Job drawing, mm, ordinate dimensions from the low corner. One solid piece. A direction names the side the tool comes from. Round coordinates to 2 decimals unless told otherwise and drop trailing zeros. Loops run counter-clockwise (first coordinate to the right, second up) from the corner with the lowest first, then second, coordinate; pieces in that order, holes last.
1) Band-saw the part on A-A, the plane x = 210. Write the cut outline in (y, z).
2) Drop flat-ended pins along their axis: P1, Ø1.5, axis at y = 9.5, z = 34, coming from the +X side; P2, Ø6, axis at x = 28, y = 4.5, coming from the +Z side; P3, Ø6, axis at x = 200.5, y = 13, coming from the -Z side. Give the stop position or say it passes through.
3) 3-axis set-ups, long thin cutter, end or side, ignore diameter. For the marked faces 4, 5 and 6: which of +Z, -Z, +X, -X, +Y, -Y reach the whole face in a straight line?
4) Band-saw the part on B-B, the plane y = 14.5. Write the cut outline in (x, z), then the cut area to 3 significant figures.
5) Band-saw the part on C-C, the plane z = 45. Write the cut outline in (x, y), then the cut area to 3 significant figures.
6) Probe line 1 (Z direction, x = 102, y = 11.5); line 2 (Z direction, x = 45, y = 10); line 3 (X direction, y = 13.25, z = 45). List the from-to ranges inside material, lowest first.
7) Mould opens along X. For the marked faces 1, 2 and 3 say: +X half, -X half, draft (parallel to the pull), parting line (faces both ways), or undercut.
8) Band-saw the part on D-D, the plane x = 45. Write the cut outline in (y, z), then the cut area to 3 significant figures.
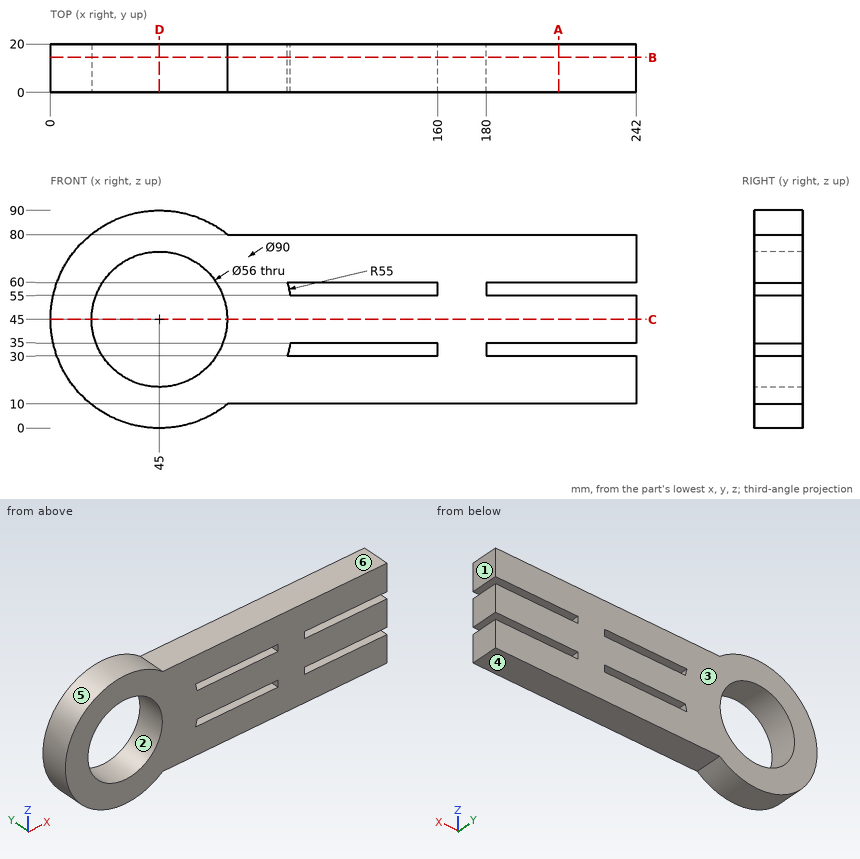
Reported:
1. outline: (0, 10) - (20, 10) - (20, 30) - (0, 30) - close; (0, 35) - (20, 35) - (20, 55) - (0, 55) - close; (0, 60) - (20, 60) - (20, 80) - (0, 80) - close
2. P1: stops at x = 180
2. P2: stops at z = 87.77
2. P3: stops at z = 10
3. face 4: -Z, +X, +Y, -Y
3. face 5: +Y, -Y
3. face 6: +Z, +X, +Y, -Y
4. outline: (73.28, 10) - (242, 10) - (242, 30) - (180, 30) - (180, 35) - (242, 35) - (242, 55) - (180, 55) - (180, 60) - (242, 60) - (242, 80) - (73.28, 80) arc R45 ccw (long way) to start; hole circle Ø56 at (45, 45); hole (97.92, 30) - (160, 30) - (160, 35) - (99.08, 35) arc R55 cw to start; hole (97.92, 60) arc R55 cw to (99.08, 55) - (160, 55) - (160, 60) - close
4. area: 13,700 mm2
5. outline: (0, 0) - (17, 0) - (17, 20) - (0, 20) - close; (73, 0) - (242, 0) - (242, 20) - (73, 20) - close
5. area: 3,720 mm2
6. line 1: z = 10 to 30, 35 to 55, 60 to 80
6. line 2: z = 0 to 17, 73 to 90
6. line 3: x = 0 to 17, 73 to 242
7. face 1: +X half
7. face 2: undercut
7. face 3: draft
8. outline: (0, 0) - (20, 0) - (20, 17) - (0, 17) - close; (0, 73) - (20, 73) - (20, 90) - (0, 90) - close
8. area: 680 mm2
